Geometry check sheet. Reference: the model listing, model coordinates, mm. Face numbers are marked on the shaded views. A direction names the side the tool comes from. Round coordinates to 2 decimals unless told otherwise and drop trailing zeros. Order: outer loops, then holes, each group sorted by start corner. A loop starts at its lowest first (then second) coordinate and runs counter-clockwise, first axis right, second up.
(1) Go/stop test with a flat-tipped pin: pin 1 (3 mm diameter, centred on x = -9.5, y = -6, fed in from +Z). Record where the tip stops, or that it passes through.
(2) Material ranges on line 1 along Y through (x, z) = (22.5, 8.75); line 2 along X through (y, z) = (0.25, 1.5); line 3 along Y through (x, z) = (-22, 0.5), recorded low to high.
(3) Release check for a two-part mould opening along X. For the marked faces 3, 4, 5 and 6 record: +X half, -X half, draft (parallel to the pull), parting line (faces both ways), or undercut.
(4) Sectioned sample at A-A (y = 9.25). Record the boundary of the cut face in (x, z).
(5) Sectioned sample at C-C (x = -22.5). Record the boundary of the cut face in (y, z), plus the area to 3 significant figures.
(6) Sectioned sample at B-B (y = -9.25). Record the boundary of the cut face in (x, z).
(7) Sectioned sample at D-D (y = 6.25). Record the boundary of the cut face in (x, z).
(8) Set-up check for the marked faces 1 and 2: record each of +Z, -Z, +X, -X, +Y, -Y from which the full face is reachable in a straight line by a thin tool's end or side.
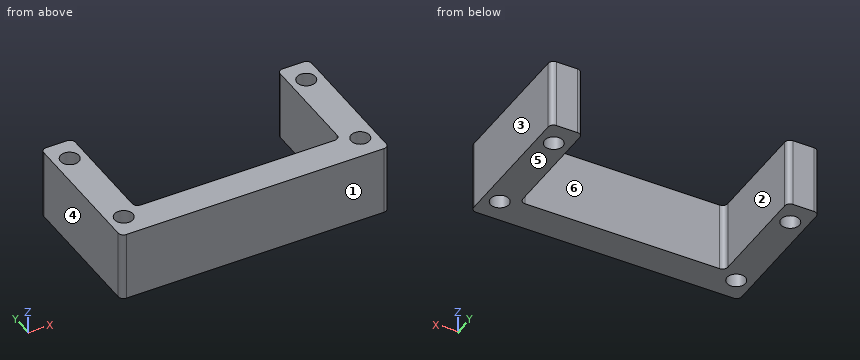
from build123d import *

# Parameters (mm, degrees)
EXTRUDE_1_DEPTH     = 13.23
SKETCH_3_R          = 1.75
CUT_EXTRUDE_2_DEPTH = 32.848789616
FILLET_1_R          = 1


with BuildPart() as part:
    # 草图1 → 凸台-拉伸1 (new body)
    with BuildSketch(Plane.XY):
        Polygon((-19.5, 13.75), (-19.5, -7.75), (19.5, -7.75), (19.5, 13.75), (25.5, 13.75), (25.5, -13.75), (-25.5, -13.75), (-25.5, 13.75), align=None)
    extrude(amount=EXTRUDE_1_DEPTH)

    # 草图3 → 切除-拉伸2 (cut, through all)
    with BuildSketch(Plane.XY.offset(13.23)):
        with Locations((-22.5, 9.25)):
            Circle(SKETCH_3_R)
        with Locations((-22.5, -9.25)):
            Circle(SKETCH_3_R)
        with Locations((22.5, -9.25)):
            Circle(SKETCH_3_R)
        with Locations((22.5, 9.25)):
            Circle(SKETCH_3_R)
    extrude(amount=-CUT_EXTRUDE_2_DEPTH, mode=Mode.SUBTRACT)

    # 圆角1
    fillet_1_edges = [part.edges().sort_by_distance(p)[0] for p in [
        (25.5, -13.75, 6.615),
        (-25.5, -13.75, 6.615),
        (-25.5, 13.75, 6.615),
        (-19.5, 13.75, 6.615),
        (-19.5, -7.75, 6.615),
        (19.5, -7.75, 6.615),
        (19.5, 13.75, 6.615),
        (25.5, 13.75, 6.615),
    ]]
    fillet(fillet_1_edges, radius=FILLET_1_R)


solid = part.part
Answer below:
1. pin 1: passes through
2. line 1: y = -13.75 to -11, -7.5 to 7.5, 11 to 13.75
2. line 2: x = -25.5 to -19.5, 19.5 to 25.5
2. line 3: y = -13.75 to -10.93, -7.57 to 7.57, 10.93 to 13.75
3. face 3: +X half
3. face 4: -X half
3. face 5: draft
3. face 6: undercut
4. outline: (-25.5, 0) - (-24.25, 0) - (-24.25, 13.23) - (-25.5, 13.23) - close; (-20.75, 0) - (-19.5, 0) - (-19.5, 13.23) - (-20.75, 13.23) - close; (19.5, 0) - (20.75, 0) - (20.75, 13.23) - (19.5, 13.23) - close; (24.25, 0) - (25.5, 0) - (25.5, 13.23) - (24.25, 13.23) - close
5. outline: (-13.75, 0) - (-11, 0) - (-11, 13.23) - (-13.75, 13.23) - close; (-7.5, 0) - (7.5, 0) - (7.5, 13.23) - (-7.5, 13.23) - close; (11, 0) - (13.75, 0) - (13.75, 13.23) - (11, 13.23) - close
5. area: 271 mm2
6. outline: (-25.5, 0) - (-24.25, 0) - (-24.25, 13.23) - (-25.5, 13.23) - close; (-20.75, 0) - (20.75, 0) - (20.75, 13.23) - (-20.75, 13.23) - close; (24.25, 0) - (25.5, 0) - (25.5, 13.23) - (24.25, 13.23) - close
7. outline: (-25.5, 0) - (-19.5, 0) - (-19.5, 13.23) - (-25.5, 13.23) - close; (19.5, 0) - (25.5, 0) - (25.5, 13.23) - (19.5, 13.23) - close
8. face 1: +Z, -Z, +X, -X, -Y
8. face 2: +Z, -Z, +Y
